Input: part model. Units: mm. Frame: model coordinates. A direction names the side the tool comes from. Coordinates: 2 decimals unless noted, no trailing zeros. Loops run counter-clockwise (first coordinate to the right, second up) from the corner with the lowest first, then second, coordinate; pieces in that order, holes last.
(1) Contact query for flat-ended pins moving along their axis: P1, Ø3.5, axis at x = -24, y = -5, coming from the +Z side; P2, Ø5.5, axis at x = -4.5, z = 5.53, coming from the -Y side; P3, Ø10.5, axis at x = 0.5, y = -1.5, coming from the +Z side. Output: stop coordinate, or through.
(2) Mould query, pull axis Y, two halves, no side actions, for faces 1 (the face through (0, -20.86, -2)), 2 (the face through (-25.65, 16.48, 8.69)), 3 (the face through (-25.5, 5.07, -1.97)). Classes: released by +Y, released by -Y, zero draft, split by the parting line, or undercut.
(3) Section B-B, the plane y = -1.5. Return loops of the section in (x, z).
(4) Section D-D, the plane y = 5. Return loops of the section in (x, z).
(5) Set-up query: faces 4 (the face through (0, 10, -2)), 5 (the face through (25.49, 16.48, 8.85)), 6 (the face through (0, -11, 0)). Return all of +Z, -Z, +X, -X, +Y, -Y with unobstructed straight access to the full face (end or side cutting, diameter ignored); none if empty.
(6) Section C-C, the plane x = -4.5. Return loops of the section in (y, z), then the cut area to 3 significant figures.
(7) Section A-A, the plane x = 4.5. Return loops of the section in (y, z), then the cut area to 3 significant figures.
(8) Line query: L1, parallel to Y at x = -24, z = -1.4; L2, parallel to Y at x = -3, z = -0.75; L3, parallel to Z at x = -3.5, y = 11. Output: solid intervals per line, ascending.
```python
from build123d import *

# Parameters (mm, degrees)
SKETCH1_W           = 57
SKETCH1_H           = 35
SKETCH1_R           = 1.5
SKETCH1_W_2         = 41
SKETCH1_H_2         = 20
BASE_FLANGE2_DEPTH  = 4
EDGE_FLANGE1_DEPTH  = 57
FILLET1_R           = 10
SKETCH22_R          = 2.35
CUT_EXTRUDE4_DEPTH  = 10
SKETCH17_W          = 57
SKETCH17_H          = 15.7
BOSS_EXTRUDE1_DEPTH = 4.7366
SKETCH25_R          = 2.35
CUT_EXTRUDE5_DEPTH  = 51.280586508
FILLET2_R           = 10


# Sheet-metal steps are written as plain solids
with BuildPart() as part:
    # Sketch1 → Base-Flange2 (new body)
    with BuildSketch(Plane.XY):
        with Locations((0, -3.36)):
            Rectangle(SKETCH1_W, SKETCH1_H)
        with Locations((-24, 5)):
            Circle(SKETCH1_R, mode=Mode.SUBTRACT)
        with Locations(Location((24, 5, 0), (0, 0, 180))):
            Circle(SKETCH1_R, mode=Mode.SUBTRACT)
        with Locations((24, -5)):
            Circle(SKETCH1_R, mode=Mode.SUBTRACT)
        with Locations(Location((-24, -5, 0), (0, 0, 180))):
            Circle(SKETCH1_R, mode=Mode.SUBTRACT)
        Rectangle(SKETCH1_W_2, SKETCH1_H_2, mode=Mode.SUBTRACT)
    extrude(amount=-BASE_FLANGE2_DEPTH)

    # Edge-Flange1 section (across the edge) → Edge-Flange1 (add)
    with BuildSketch(Plane(origin=(28.5, 14.8766, 0), x_dir=(0, -1, 0), z_dir=(-1, 0, 0))):
        with BuildLine():
            Line((-4, 0.7366), (-4, 11.7))
            Line((-4, 11.7), (0, 11.7))
            Line((0, 11.7), (0, 0.7366))
            ThreePointArc((0, 0.7366), (0.215745145, 0.215745145), (0.7366, 0))
            Line((0.7366, 0), (0.7366, -4))
            ThreePointArc((0.7366, -4), (-2.61268198, -2.61268198), (-4, 0.7366))
        make_face()
    extrude(amount=EDGE_FLANGE1_DEPTH)

    # Fillet1
    fillet1_edges = [part.edges().sort_by_distance(p)[0] for p in [
        (28.5, 16.8766, 11.7),
        (-28.5, 16.8766, 11.7),
        (28.5, -20.86, -2),
        (-28.5, -20.86, -2),
    ]]
    fillet(fillet1_edges, radius=FILLET1_R)

    # Sketch22 → Cut-Extrude4 (cut)
    with BuildSketch(Plane(origin=(0, 18.8766, 0), x_dir=(1, 0, 0), z_dir=(0, 1, 0))):
        with Locations(Location((-4.5, -5.521282453, 0), (0, 0, 270))):
            Circle(SKETCH22_R)
        with Locations(Location((10.5, -5.521282453, 0), (0, 0, 270))):
            Circle(SKETCH22_R)
    extrude(amount=-CUT_EXTRUDE4_DEPTH, mode=Mode.SUBTRACT)

    # Sketch17 → Boss-Extrude1 (add)
    with BuildSketch(Plane(origin=(0, 18.8766, 0), x_dir=(1, 0, 0), z_dir=(0, 1, 0))):
        with Locations((0, -3.85)):
            Rectangle(SKETCH17_W, SKETCH17_H)
    extrude(amount=-BOSS_EXTRUDE1_DEPTH)

    # Sketch25 → Cut-Extrude5 (cut, through all)
    with BuildSketch(Plane(origin=(0, 18.8766, 0), x_dir=(1, 0, 0), z_dir=(0, 1, 0))):
        with Locations(Location((-4.5, -5.53, 0), (0, 0, 270))):
            Circle(SKETCH25_R)
        with Locations(Location((10.5, -5.53, 0), (0, 0, 270))):
            Circle(SKETCH25_R)
    extrude(amount=-CUT_EXTRUDE5_DEPTH, mode=Mode.SUBTRACT)

    # Fillet2
    fillet2_edges = [part.edges().sort_by_distance(p)[0] for p in [
        (-28.5, 16.5083, 11.7),
        (28.5, 16.5083, 11.7),
    ]]
    fillet(fillet2_edges, radius=FILLET2_R)


solid = part.part
```
Report:
1. P1: stops at z = 0
1. P2: stops at y = 14.14
1. P3: passes through
2. face 1: released by -Y
2. face 2: zero draft
2. face 3: undercut
3. outline: (-28.5, -4) - (-20.5, -4) - (-20.5, 0) - (-28.5, 0) - close; (20.5, -4) - (28.5, -4) - (28.5, 0) - (20.5, 0) - close
4. outline: (-28.5, -4) - (-25.5, -4) - (-25.5, 0) - (-28.5, 0) - close; (-22.5, -4) - (-20.5, -4) - (-20.5, 0) - (-22.5, 0) - close; (20.5, -4) - (22.5, -4) - (22.5, 0) - (20.5, 0) - close; (25.5, -4) - (28.5, -4) - (28.5, 0) - (25.5, 0) - close
5. face 4: +Z, -Z
5. face 5: +Z, +X, +Y, -Y
5. face 6: +Z, +X, -X, -Y
6. outline: (-20.86, -4) - (-10, -4) - (-10, 0) - (-20.86, 0) - close; (10, -4) - (18.88, -4) - (18.88, 3.18) - (14.14, 3.18) - (14.14, 0) - (10, 0) - close; (14.14, 7.88) - (18.88, 7.88) - (18.88, 11.7) - (14.14, 11.7) - close
6. area: 112 mm2
7. outline: (-20.86, -4) - (-10, -4) - (-10, 0) - (-20.86, 0) - close; (10, -4) - (18.88, -4) - (18.88, 11.7) - (14.14, 11.7) - (14.14, 0) - (10, 0) - close
7. area: 134 mm2
8. L1: y = -19.21 to -6.5, -3.5 to 3.5, 6.5 to 18.88
8. L2: y = -20.86 to -10, 10 to 18.88
8. L3: z = -4 to 0
